Model file for the job. Use its own axes, mm. Face numbers are marked on the shaded views. Coordinates: 2 decimals unless noted, no trailing zeros. Write each loop counter-clockwise with the first axis right and the second up, starting at its lowest first coordinate (ties: lowest second). Pieces come first, ordered by that corner, then holes. Notation, with made-up numbers: (-38.5, 7) - (19.5, 7) arc R20 ccw to (19.5, 32) - close; hole circle Ø6 at (-14.5, -3). An arc over 180 degrees is marked (long way). Put each result on its own line as item: value. Start each with the question number.
1. Saw through at D-D, the plane y = 6.75. Write the cut outline in (x, z), plus the area to 3 significant figures.
2. Drop a flat-ended pin along its axis: P1, Ø4, axis at x = 7.62, z = 2.54, coming from the -Y side. Give the stop position or say it passes through.
3. Saw through at C-C, the plane z = -6.5. Write the cut outline in (x, y).
4. Drill centre lines: L1, parallel to X at y = 6.75, z = 2.54; L2, parallel to X at y = 5.5, z = 2.54; L3, parallel to Z at x = -7.75, y = 7.5. Where is each one in solid material? Low to high. Write a range as from..to.
5. Saw through at A-A, the plane z = 2.54. Write the cut outline in (x, y), plus the area to 3 significant figures.
6. Pull direction Z, two halves, no side cores. Call the marked faces 1, 2 and 3: released by +Z, released by -Z, zero draft, split by the parting line, or undercut.
7. Saw through at B-B, the plane x = -7.62. Write the cut outline in (y, z).
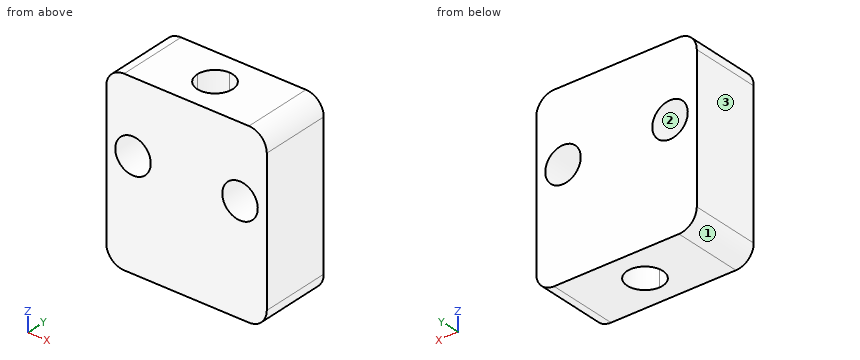
```python
from build123d import *

# Parameters (mm, degrees)
SKETCH1_W           = 22.86
SKETCH1_H           = 25.4
SKETCH1_R           = 2.5273
BOSS_EXTRUDE1_DEPTH = 10
FILLET1_R           = 2.54
CUT_EXTRUDE1_DEPTH  = 30.594001081


with BuildPart() as part:
    # Sketch1 → Boss-Extrude1 (new body)
    with BuildSketch(Plane(origin=(0, 0, 0), x_dir=(1, 0, 0), z_dir=(0, 1, 0))):
        Rectangle(SKETCH1_W, SKETCH1_H)
        with Locations(Location((-7.62, -2.54, 0), (0, 0, 270))):
            Circle(SKETCH1_R, mode=Mode.SUBTRACT)
        with Locations(Location((7.62, -2.54, 0), (0, 0, 270))):
            Circle(SKETCH1_R, mode=Mode.SUBTRACT)
    extrude(amount=BOSS_EXTRUDE1_DEPTH)

    # Fillet1
    fillet1_edges = [part.edges().sort_by_distance(p)[0] for p in [
        (11.43, 5, 12.7),
        (-11.43, 5, 12.7),
        (-11.43, 5, -12.7),
        (11.43, 5, -12.7),
    ]]
    fillet(fillet1_edges, radius=FILLET1_R)

    # Sketch4 → Cut-Extrude1 (cut, through all)
    with BuildSketch(Plane(origin=(0, 0, 12.7), x_dir=(-1, 0, 0), z_dir=(0, 0, -1))):
        with BuildLine():
            ThreePointArc((0, 7.5273), (-2.5273, 5), (0, 2.4727))
            Line((0, 2.4727), (0, 7.5273))
        make_face()
        with BuildLine():
            Line((0, 7.5273), (0, 2.4727))
            ThreePointArc((0, 2.4727), (1.787070968, 3.212929032), (2.5273, 5))
            ThreePointArc((2.5273, 5), (1.787070968, 6.787070968), (0, 7.5273))
        make_face()
    extrude(amount=CUT_EXTRUDE1_DEPTH, mode=Mode.SUBTRACT)


solid = part.part
```
Final values:
1. outline: (-11.43, -10.16) arc R2.54 ccw to (-8.89, -12.7) - (-1.82, -12.7) - (-1.82, 12.7) - (-8.89, 12.7) arc R2.54 ccw to (-11.43, 10.16) - close; (1.82, -12.7) - (8.89, -12.7) arc R2.54 ccw to (11.43, -10.16) - (11.43, 10.16) arc R2.54 ccw to (8.89, 12.7) - (1.82, 12.7) - close; hole circle Ø5.05 at (-7.62, 2.54); hole circle Ø5.05 at (7.62, 2.54)
1. area: 442 mm²
2. P1: passes through
3. outline: (-11.43, 0) - (11.43, 0) - (11.43, 10) - (-11.43, 10) - close; hole circle Ø5.05 at (0, 5)
4. L1: x = -11.43..-10.15, -5.09..-1.82, 1.82..5.09, 10.15..11.43
4. L2: x = -11.43..-10.15, -5.09..-2.48, 2.48..5.09, 10.15..11.43
4. L3: z = -12.7..0.02, 5.06..12.7
5. outline: (-11.43, 0) - (-10.15, 0) - (-10.15, 10) - (-11.43, 10) - close; (-5.09, 0) - (5.09, 0) - (5.09, 10) - (-5.09, 10) - close; (10.15, 0) - (11.43, 0) - (11.43, 10) - (10.15, 10) - close; hole circle Ø5.05 at (0, 5)
5. area: 107 mm²
6. face 1: released by -Z
6. face 2: undercut
6. face 3: zero draft
7. outline: (0, -12.7) - (10, -12.7) - (10, 0.01) - (0, 0.01) - close; (0, 5.07) - (10, 5.07) - (10, 12.7) - (0, 12.7) - close
